```python
from build123d import *

# Parameters (mm, degrees)
F1_DEPTH = 25
F2_DEPTH = 25
F3_DEPTH = 25
F4_DEPTH = 25
F5_DEPTH = 25


with BuildPart() as f1:
    # F0 (on Right) → F1 (new body)
    with BuildSketch(Plane.YZ):
        Polygon((0, 57), (0, 0), (12, 0), (12, 70), (0, 70), (0, 60), (3, 60), (3, 57), align=None)
    extrude(amount=F1_DEPTH)

    # F2 (add): a face of the model
    f2_faces = [f1.faces().sort_by_distance(p)[0] for p in [
        (25, 6.0487364621, 34.7454873646),
    ]]
    extrude(f2_faces, amount=F2_DEPTH)

    # F3 (add): a face of the model
    f3_faces = [f1.faces().sort_by_distance(p)[0] for p in [
        (50, 6.0487364621, 34.7454873646),
    ]]
    extrude(f3_faces, amount=F3_DEPTH)

    # F4 (add): a face of the model
    f4_faces = [f1.faces().sort_by_distance(p)[0] for p in [
        (75, 6.0487364621, 34.7454873646),
    ]]
    extrude(f4_faces, amount=F4_DEPTH)

    # F5 (add): a face of the model
    f5_faces = [f1.faces().sort_by_distance(p)[0] for p in [
        (100, 6.0487364621, 34.7454873646),
    ]]
    extrude(f5_faces, amount=F5_DEPTH)


solid = f1.part
```
Check sheet for the modelled part. Datum: model origin and axes. Units: mm. A direction names the side the tool comes from. Round coordinates to 2 decimals unless told otherwise and drop trailing zeros. Answer as a JSON object with one key per item and string values. Group by question number.
Q1. Gauge pin test, flat end, axial feed: P1, Ø1.5, axis at x = 39.5, z = 58, coming from the -Y side. Record the tip position at first contact, or that the pin passes through.
Q2. Set-up check for faces 1 (the face through (0, 6, 35)), 2 (the face through (62, 1, 60)): record each of +Z, -Z, +X, -X, +Y, -Y from which the full face is reachable in a straight line by a thin tool's end or side.
Q3. Scan line: line 1 along Z through (x, y) = (105, 2.5). Record every from-to range of solid material in increasing order. Write a range as [from, to].
Q4. Mould release check, pull along Z, two halves, no side actions. Record for faces 3 (the face through (62, 6, 0)), 4 (the face through (62, 2, 57)), 5 (the face through (62, 12, 35)): released by +Z, released by -Z, zero draft, split by the parting line, or undercut.
Solution:
{
 "1": {"P1": "stops at y = 3"},
 "2": {"face 1": "+Z, -Z, -X, +Y, -Y", "face 2": "+X, -X, -Y"},
 "3": {"line 1": "z = [0, 57], [60, 70]"},
 "4": {"face 3": "released by -Z", "face 4": "undercut", "face 5": "zero draft"}
}
